Job drawing, mm, ordinate dimensions from the low corner. One solid piece. A direction names the side the tool comes from. Round coordinates to 2 decimals unless told otherwise and drop trailing zeros. Write each loop counter-clockwise with the first axis right and the second up, starting at its lowest first coordinate (ties: lowest second). Pieces come first, ordered by that corner, then holes.
1) Saw through at A-A (z = 18). Write the cut outline in (x, y), plus the area to 3 significant figures.
2) Wall check: probe 1 along X at (y, z) = (365, 94.5); probe 2 along Z at (x, y) = (67, 24.5); probe 3 along Y at (x, z) = (566.5, 32.5). Give the ranges that are in metal, low to high.
3) Pull direction X, two halves, no side cores. Call the marked faces 1, 2 and 3: +X half, -X half, draft (parallel to the pull), parting line (faces both ways), or undercut.
4) Saw through at C-C (z = 91.5). State how many separate pieces and enclosed holes the cut face has, plus the area to 3 significant figures.
5) Flat gauge pins, fed straight in: pin 1 (10 mm diameter, centred on x = 183, y = 337.5, fed in from +Z); pin 2 (23.5 mm diameter, centred on y = 36, z = 113, fed in from -X). Where does each tip first touch, or does it go through?
6) Saw through at B-B (x = 190). Write the cut outline in (y, z).
7) Saw through at D-D (y = 262). Write the cut outline in (x, z) (1 decimal), plus the area to 3 significant figures.
8) Which spindle directions (+Z, -Z, +X, -X, +Y, -Y) get a long thin tool onto all of the face, cutting with end or side? Do the marked faces 4 and 5. Say none if no direction does.
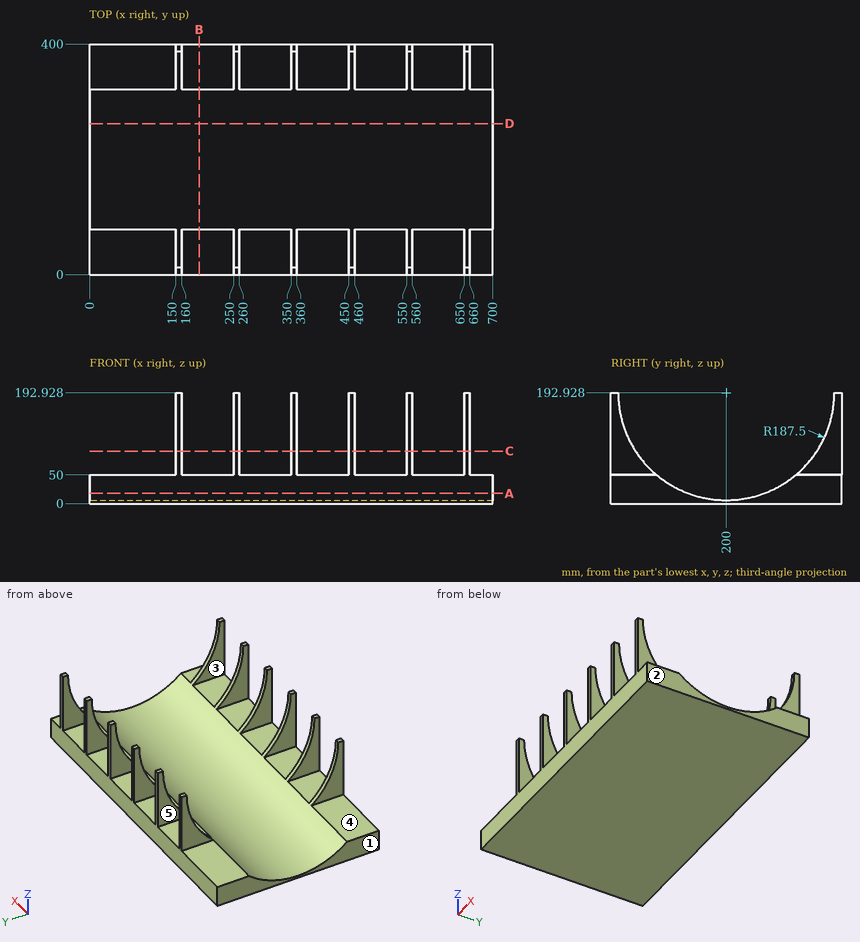
Evaluation:
1. outline: (0, 0) - (700, 0) - (700, 132.5) - (0, 132.5) - close; (0, 267.5) - (700, 267.5) - (700, 400) - (0, 400) - close
1. area: 185,000 mm2
2. probe 1: x = 150 to 160, 250 to 260, 350 to 360, 450 to 460, 550 to 560, 650 to 660
2. probe 2: z = 0 to 50
2. probe 3: y = 0 to 102.95, 297.05 to 400
3. face 1: -X half
3. face 2: +X half
3. face 3: undercut
4. separate pieces: 12
4. enclosed holes: 0
4. area: 5,080 mm2
5. pin 1: stops at z = 50
5. pin 2: stops at x = 150
6. outline: (0, 0) - (400, 0) - (400, 50) - (321.36, 50) arc R187.5 cw to (78.64, 50) - (0, 50) - close
7. outline: (0, 0) - (700, 0) - (700, 16) - (0, 16) - close
7. area: 11,200 mm2
8. face 4: +Z, -X, +Y, -Y
8. face 5: +Z, +Y, -Y
